```python
from build123d import *

# Parameters (mm, degrees)
SKETCH1_R                       = 12.573
BOSS_EXTRUDE1_DEPTH             = 13.716
SKETCH2_R                       = 7.62
CUT_EXTRUDE1_DEPTH              = 10.16
F_1_8_0_1250_DOWEL_HOLE1_REACH  = 31.128
F_1_8_0_1250_DOWEL_HOLE1_BORE_R = 1.5875
CUT_EXTRUDE3_DEPTH              = 10
CUT_EXTRUDE3_DEPTH_BACK         = 10.16
CIRPATTERN1_COUNT               = 4


with BuildPart() as part:
    # Sketch1 → Boss-Extrude1 (new body)
    with BuildSketch(Plane.XY):
        Circle(SKETCH1_R)
    extrude(amount=BOSS_EXTRUDE1_DEPTH)

    # Sketch2 → Cut-Extrude1 (cut)
    with BuildSketch(Plane.XY.offset(13.716)):
        Circle(SKETCH2_R)
    extrude(amount=-CUT_EXTRUDE1_DEPTH, mode=Mode.SUBTRACT)

    # 1/8 (0.1250) Dowel Hole1 bore → 1/8 (0.1250) Dowel Hole1 (cut, up to next)
    with BuildSketch(Plane(origin=(0, 12.573, 7.62), x_dir=(1, 0, 0), z_dir=(0, 1, 0)), mode=Mode.PRIVATE) as f_1_8_0_1250_dowel_hole1_sk1:
        with Locations((0, 0.014313547)):
            Circle(F_1_8_0_1250_DOWEL_HOLE1_BORE_R)
    f_1_8_0_1250_dowel_hole1_tool1 = extrude(f_1_8_0_1250_dowel_hole1_sk1.sketch, amount=-F_1_8_0_1250_DOWEL_HOLE1_REACH, mode=Mode.PRIVATE) & part.part
    add(f_1_8_0_1250_dowel_hole1_tool1.solids().sort_by_distance((0, 12.573, 7.605686))[0], mode=Mode.SUBTRACT)

    # Sketch5 → Cut-Extrude3 (cut, two sides)
    with BuildSketch(Plane(origin=(0, 0, 7.62), x_dir=(-1, 0, 0), z_dir=(0, 0, -1))) as cut_extrude3_sk:
        with BuildLine():
            Line((1.5, 1.99598875), (-1.5, 1.99598875))
            ThreePointArc((-1.5, 1.99598875), (-1.118033989, -2.240079228), (2.5, -0.00401125))
            ThreePointArc((2.5, -0.00401125), (2.236067977, 1.114022739), (1.5, 1.99598875))
        make_face()
    extrude(amount=CUT_EXTRUDE3_DEPTH, mode=Mode.SUBTRACT)
    extrude(cut_extrude3_sk.sketch, amount=-CUT_EXTRUDE3_DEPTH_BACK, mode=Mode.SUBTRACT)

    # Sketch15 → #2-56 Tapped Hole1 (revolve, cut)
    with BuildSketch(Plane(origin=(7.184204897, -7.188216147, 13.716), x_dir=(0, -1, 0), z_dir=(1, 0, 0))):
        Polygon((0, 0), (0, 8.24814509), (0.889, 7.71398), (0.889, 0), align=None)
    f_2_56_tapped_hole1 = revolve(axis=Axis((7.184204897, -7.188216147, 20.066), (0, 0, -1)), mode=Mode.SUBTRACT)

    # CirPattern1: #2-56 Tapped Hole1 ×4 about axis
    cirpattern1_axis = Axis((0, -0.00401125, 0), (0, 0, 1))
    for i in range(1, CIRPATTERN1_COUNT):
        add(f_2_56_tapped_hole1.rotate(cirpattern1_axis, i * 360 / CIRPATTERN1_COUNT), mode=Mode.SUBTRACT)


solid = part.part
```
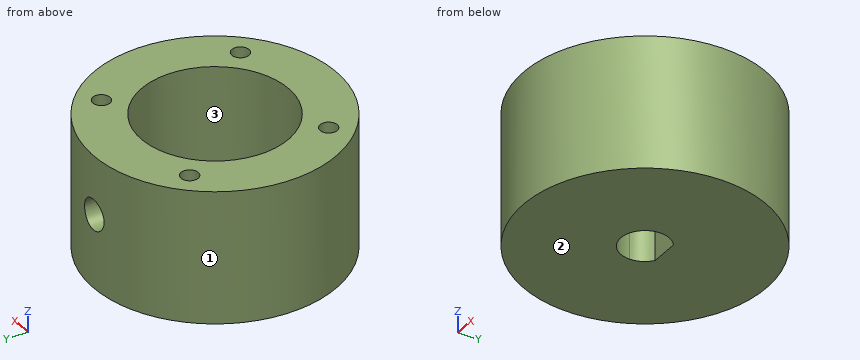
Build history of the part. All positions in model axes, mm. Face numbers are marked on the shaded views. Give positions to 0.01 mm unless a question says otherwise; leave off trailing zeros. Loops run counter-clockwise (first coordinate to the right, second up) from the corner with the lowest first, then second, coordinate; pieces in that order, holes last.
1) Band-saw the part on D-D on y = 4.5. List the corners of the cut face in (x, z).
Values follow:
outline: (-11.74, 0) - (11.74, 0) - (11.74, 13.72) - (6.15, 13.72) - (6.15, 3.56) - (-6.15, 3.56) - (-6.15, 13.72) - (-11.74, 13.72) - close
2) Drop flat-ended pins along their axis: P1, Ø1.4, axis at x = 7.18, y = 7.18, coming from the +Z side; P2, Ø1.1, axis at x = 7.18, y = -7.19, coming from the -Z side; P3, Ø1, axis at x = 0.5, y = 0, coming from the +Z side; P4, Ø2, axis at x = -0.5, y = -2, coming from the +Z side. Give the stop position or say it passes through.
Values follow:
P1: stops at z = 5.89
P2: stops at z = 0
P3: passes through
P4: stops at z = 3.56
3) Band-saw the part on C-C on z = 9.75. List the corners of the cut face in (x, y), then the cut area to 3 significant figures.
Values follow:
outline: circle Ø25.15 at (0, 0); hole circle Ø1.78 at (-7.18, -7.19); hole circle Ø1.78 at (-7.18, 7.18); hole circle Ø15.24 at (0, 0); hole circle Ø1.78 at (7.18, -7.19); hole circle Ø1.78 at (7.18, 7.18)
area: 304 mm2
4) Band-saw the part on B-B on y = -1. List the corners of the cut face in (x, z), then the cut area to 3 significant figures.
Values follow:
outline: (-12.53, 0) - (-2.29, 0) - (-2.29, 3.56) - (-7.55, 3.56) - (-7.55, 13.72) - (-12.53, 13.72) - close; (2.29, 0) - (12.53, 0) - (12.53, 13.72) - (7.55, 13.72) - (7.55, 3.56) - (2.29, 3.56) - close
area: 174 mm2
5) Probe line 1 along Y through (x, z) = (0, 11.5); line 2 along Z through (x, y) = (0, 10.95); line 3 along X through (y, z) = (-7, 10.5). List the from-to ranges inside material, lowest first.
Values follow:
line 1: y = -12.57 to -7.62, 7.62 to 12.57
line 2: z = 0 to 6.02, 9.19 to 13.72
line 3: x = -10.44 to -8.05, -6.32 to -3.01, 3.01 to 6.32, 8.05 to 10.44
6) Band-saw the part on A-A on x = 0. List the corners of the cut face in (y, z), then the cut area to 3 significant figures.
Values follow:
outline: (-12.57, 0) - (-2.5, 0) - (-2.5, 3.56) - (-7.62, 3.56) - (-7.62, 13.72) - (-12.57, 13.72) - close; (2, 0) - (12.57, 0) - (12.57, 6.02) - (7.62, 6.02) - (7.62, 3.56) - (2, 3.56) - close; (7.62, 9.19) - (12.57, 9.19) - (12.57, 13.72) - (7.62, 13.72) - close
area: 158 mm2
7) Two-plate mould, pull along X, no slides. Class the marked faces 1, 2 and 3: released by +X, released by -X, zero draft, split by the parting line, or undercut.
Values follow:
face 1: split by the parting line
face 2: zero draft
face 3: undercut
